Geometry: see drawing. Coordinates: mm, zero at the bounding-box minimum. Give positions to 0.01 mm unless a question says otherwise; leave off trailing zeros. Write each loop counter-clockwise with the first axis right and the second up, starting at its lowest first coordinate (ties: lowest second). Pieces come first, ordered by that corner, then holes. Notation, with made-up numbers: (-14.75, 66.5) - (36.25, 66.5) arc R33 ccw to (36.25, 104.5) - close; hole circle Ø3 at (60, 87). An arc over 180 degrees is marked (long way). One line per question, with ' | ' between items. Start each with the question number.
(1) Section B-B, the plane y = 12.5. Return loops of the section in (x, z).
(2) Section A-A, the plane x = 12.5. Return loops of the section in (y, z).
(3) Draft query along X for the marked faces 1, 2, 3 and 4. Return one class per face: +X half, -X half, draft (parallel to the pull), parting line (faces both ways), or undercut.
(4) Pin query (flat end, axial travel): pin 1 (1 mm diameter, centred on y = 15, z = 3.5, fed in from -X). Return the tip coordinate at first contact, or that it passes through.
(5) Ray query, line 1 (Y direction, x = 12.5, z = 2.25); line 2 (X direction, y = 12.5, z = 4.25); line 3 (Y direction, x = 15, z = 3). Return the intervals inside material, ascending. Write a range as [from, to].
(6) Section C-C, the plane z = 7.25. Return loops of the section in (x, y).
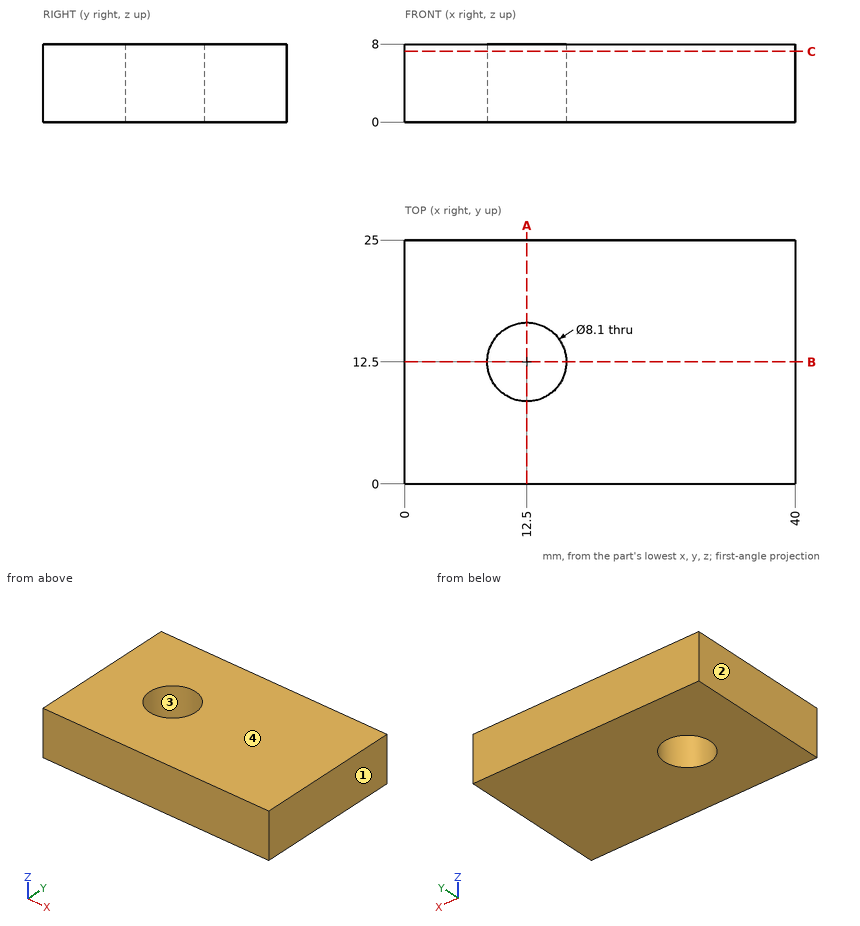
Check sheet entries:
1) outline: (0, 0) - (8.45, 0) - (8.45, 8) - (0, 8) - close; (16.55, 0) - (40, 0) - (40, 8) - (16.55, 8) - close
2) outline: (0, 0) - (8.45, 0) - (8.45, 8) - (0, 8) - close; (16.55, 0) - (25, 0) - (25, 8) - (16.55, 8) - close
3) face 1: +X half | face 2: -X half | face 3: undercut | face 4: draft
4) pin 1: x = 0
5) line 1: [0, 8.45], [16.55, 25] | line 2: [0, 8.45], [16.55, 40] | line 3: [0, 9.31], [15.69, 25]
6) outline: (0, 0) - (40, 0) - (40, 25) - (0, 25) - close; hole circle Ø8.1 at (12.5, 12.5)
